Could you check a few things on this drawing? It's one solid part, dimensions in mm from its lowest x, y, z. A direction names the side the tool comes from. Give positions to 0.01 mm unless a question says otherwise; leave off trailing zeros. Loops run counter-clockwise (first coordinate to the right, second up) from the corner with the lowest first, then second, coordinate; pieces in that order, holes last. Notation, with made-up numbers: (37, 47.25) - (42, 47.25) arc R19 ccw to (42, 83.25) - close; hole circle Ø1 at (87.5, 83.5). An arc over 180 degrees is marked (long way). Answer as a JSON object with one key per item and string values.
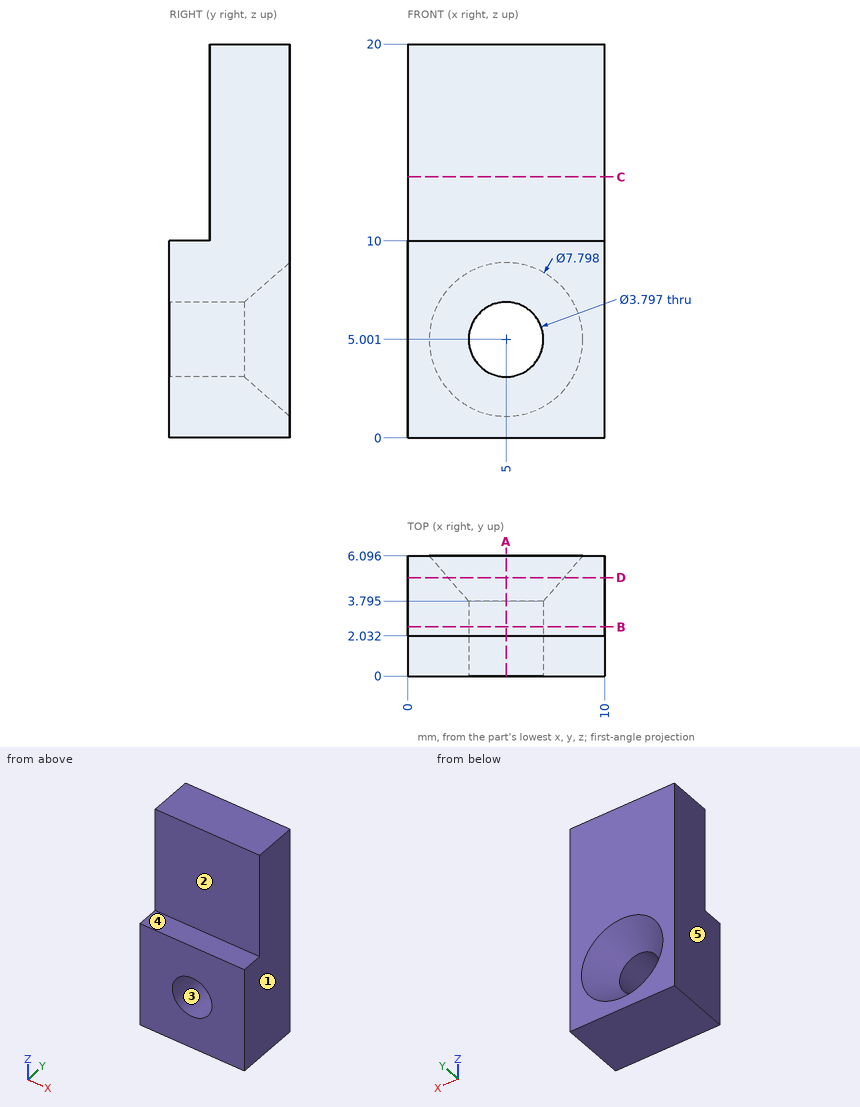
1) Imagine slicing it at D-D on y = 5. Write out the boundary of the cut face in (x, z), and give its area (3 significant figures).
Check sheet entries:
{"outline": "(0, 0) - (10, 0) - (10, 20) - (0, 20) - close; hole circle Ø5.89 at (5, 5)", "area": "173 mm2"}
2) Imagine slicing it at B-B on y = 2.5. Write out the boundary of the cut face in (x, z), and give its area (3 significant figures).
Check sheet entries:
{"outline": "(0, 0) - (10, 0) - (10, 20) - (0, 20) - close; hole circle Ø3.8 at (5, 5)", "area": "189 mm2"}
3) Imagine slicing it at A-A on x = 5. Write out the boundary of the cut face in (y, z) (1 decimal).
Check sheet entries:
{"outline": "(0, 0) - (6.1, 0) - (6.1, 1.1) - (3.8, 3.1) - (0, 3.1) - close; (0, 6.9) - (3.8, 6.9) - (6.1, 8.9) - (6.1, 20) - (2, 20) - (2, 10) - (0, 10) - close"}
4) I need wall thicknesses on L1, parallel to Z at x = 5, y = 2.6; L2, parallel to Z at x = 5, y = 1.25; L3, parallel to Y at x = 8.5, z = 19.25. Which ranges of each line are inside material? Lowest first, please.
Check sheet entries:
{"L1": "0 to 3.1, 6.9 to 20", "L2": "0 to 3.1, 6.9 to 10", "L3": "2.03 to 6.1"}
5) If we mould it in two halves opening along X, with no side actions, what happens to the marked faces 3, 4 and 5? For each: released by +X, released by -X, zero draft, split by the parting line, or undercut.
Check sheet entries:
{"face 3": "undercut", "face 4": "zero draft", "face 5": "released by -X"}
6) I'm going to push flat-ended pins straight in: P1, Ø3, axis at x = 5, z = 5, coming from the -Y side; P2, Ø2, axis at x = 3, y = 0.5, coming from the +Z side; P3, Ø5, axis at x = 3.5, z = 14.5, coming from the -Y side. Where does each tip first touch, or does it pass through?
Check sheet entries:
{"P1": "through", "P2": "z = 10", "P3": "y = 2.03"}
7) Imagine slicing it at C-C on z = 13.25. Write out the boundary of the cut face in (x, y).
Check sheet entries:
{"outline": "(0, 2.03) - (10, 2.03) - (10, 6.1) - (0, 6.1) - close"}
8) Which directions (+Z, -Z, +X, -X, +Y, -Y) give clear straight access to the entire face, cutting with the end or side of a thin tool? Please do the marked faces 1 and 2.
Check sheet entries:
{"face 1": "+Z, -Z, +X, +Y, -Y", "face 2": "+Z, +X, -X, -Y"}
